from build123d import *

# Parameters (mm, degrees)
F0_W     = 152.4
F0_H     = 152.4
F1_DEPTH = 101.6
F2_T     = -2.54
F3_R     = 5.08
F4_DEPTH = 149.86
F5_W     = 27.94
F5_H     = 50.8
F6_DEPTH = 63.5
F7_R     = 12.954
F8_DEPTH = 50.8
F9_R     = 12.7
F10_R    = 12.7


with BuildPart() as f1:
    # F0 (on Top) → F1 (new body)
    with BuildSketch(Plane.XY):
        Rectangle(F0_W, F0_H)
    extrude(amount=F1_DEPTH)

    # F2
    f2_openings = [f1.faces().sort_by_distance(p)[0] for p in [
        (0, 0, 101.6),
    ]]
    offset(amount=F2_T, openings=f2_openings)

    # F3 (on face) → F4 (join)
    with BuildSketch(Plane(origin=(0, -73.66, 0), x_dir=(-1, 0, 0), z_dir=(0, 1, 0))):
        with Locations((-35.56, 40.64)):
            Circle(F3_R)
    extrude(amount=F4_DEPTH)

    # F5 (on face) → F6 (join)
    with BuildSketch(Plane.XY.offset(2.54)):
        Rectangle(F5_W, F5_H)
    extrude(amount=F6_DEPTH)

    # F7 (on face) → F8 (cut)
    with BuildSketch(Plane(origin=(0, 25.4, 0), x_dir=(-1, 0, 0), z_dir=(0, 1, 0))):
        with Locations((0, 34.29)):
            Circle(F7_R)
    extrude(amount=-F8_DEPTH, mode=Mode.SUBTRACT)

    # F9
    f9_edges = [f1.edges().sort_by_distance(p)[0] for p in [
        (-13.97, 0, 66.04),
    ]]
    fillet(f9_edges, radius=F9_R)

    # F10
    f10_edges = [f1.edges().sort_by_distance(p)[0] for p in [
        (13.97, 0, 66.04),
    ]]
    fillet(f10_edges, radius=F10_R)


solid = f1.part
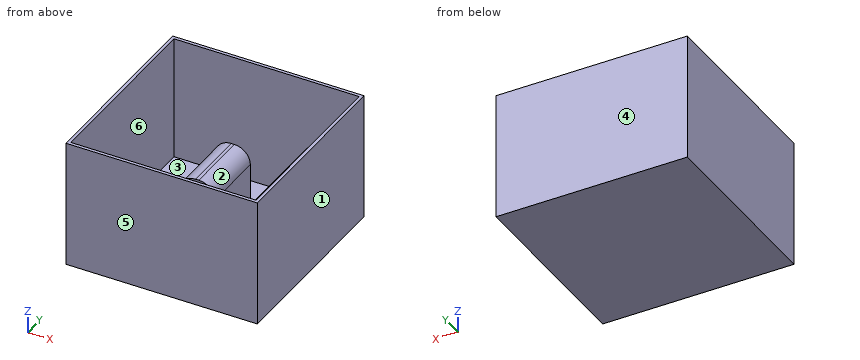
Check sheet for the modelled part. Datum: model origin and axes. Units: mm. Face numbers are marked on the shaded views. A direction names the side the tool comes from. Give positions to 0.01 mm unless a question says otherwise; leave off trailing zeros. Write each loop counter-clockwise with the first axis right and the second up, starting at its lowest first coordinate (ties: lowest second). Pieces come first, ordered by that corner, then holes. Notation, with made-up numbers: (61, -2) -> (93, -2) arc R19 cw to (93, 4) -> close; hole circle Ø3 at (45, 61.5). An arc over 180 degrees is marked (long way). Write item = value, one per line.
Item 1: Tool access check on the marked faces 5 and 6. Record the directions out of +Z, -Z, +X, -X, +Y, -Y that give a thin tool (end or side, any length) a straight path to the whole face; none if there is none.
Output:
face_5 = +Z, -Z, +X, -X, -Y
face_6 = +Z
Item 2: Sectioned sample at A-A on z = 50.5. Record the boundary of the cut face in (x, y).
Output:
outline = (-76.2, -76.2) -> (76.2, -76.2) -> (76.2, 76.2) -> (-76.2, 76.2) -> close; (-13.97, -25.4) -> (13.97, -25.4) -> (13.97, 25.4) -> (-13.97, 25.4) -> close; hole (-73.66, -73.66) -> (73.66, -73.66) -> (73.66, 73.66) -> (-73.66, 73.66) -> close
Item 3: Sectioned sample at D-D on x = 35.56. Record the boundary of the cut face in (y, z), and give its area (3 significant figures).
Output:
outline = (-76.2, 0) -> (76.2, 0) -> (76.2, 101.6) -> (73.66, 101.6) -> (73.66, 45.72) -> (-73.66, 45.72) -> (-73.66, 101.6) -> (-76.2, 101.6) -> close; hole (-73.66, 2.54) -> (73.66, 2.54) -> (73.66, 35.56) -> (-73.66, 35.56) -> close
area = 2,390 mm^2
Item 4: Scan lines: probe 1 along Y at (x, z) = (12, 20); probe 2 along X at (y, z) = (-12, 34); probe 3 along X at (y, z) = (21, 19.5). Record each from-to range of solid material in increasing order. Write a range as from..to.
Output:
probe_1 = -76.2..-73.66, -25.4..25.4, 73.66..76.2
probe_2 = -76.2..-73.66, -13.97..-12.95, 12.95..13.97, 73.66..76.2
probe_3 = -76.2..-73.66, -13.97..13.97, 73.66..76.2
Item 5: Sectioned sample at C-C on x = 62. Record the boundary of the cut face in (y, z).
Output:
outline = (-76.2, 0) -> (76.2, 0) -> (76.2, 101.6) -> (73.66, 101.6) -> (73.66, 2.54) -> (-73.66, 2.54) -> (-73.66, 101.6) -> (-76.2, 101.6) -> close
Item 6: Release check for a two-part mould opening along Y. For the marked faces 1, 2, 3 and 4 record: +Y half, -Y half, draft (parallel to the pull), parting line (faces both ways), or undercut.
Output:
face_1 = draft
face_2 = undercut
face_3 = undercut
face_4 = +Y half
Item 7: Gauge pin test, flat ends, axial feed: pin 1 (1 mm diameter, centred on x = -20, y = -59, fed in from +Z); pin 2 (2 mm diameter, centred on x = 0, y = -1, fed in from +Z); pin 3 (2 mm diameter, centred on x = -31, y = -47, fed in from -Z). Record the tip position at first contact, or that the pin passes through.
Output:
pin_1 = 2.54
pin_2 = 66.04
pin_3 = 0
Item 8: Sectioned sample at B-B on y = -54.5. Record the boundary of the cut face in (x, z).
Output:
outline = (-76.2, 0) -> (76.2, 0) -> (76.2, 101.6) -> (73.66, 101.6) -> (73.66, 2.54) -> (-73.66, 2.54) -> (-73.66, 101.6) -> (-76.2, 101.6) -> close; circle Ø10.16 at (35.56, 40.64)
